Check sheet for the modelled part. Datum: model origin and axes. Units: mm. A direction names the side the tool comes from. Give positions to 0.01 mm unless a question says otherwise; leave off trailing zeros. Order: outer loops, then holes, each group sorted by start corner. A loop starts at its lowest first (then second) coordinate and runs counter-clockwise, first axis right, second up. Notation, with made-up numbers: (76.25, 55) -> (129.25, 55) arc R20 ccw to (129.25, 76) -> close; hole circle Ø10 at (55, -29). An arc over 180 degrees is marked (long way). One line per question, with ' | ' between items. Start each with the question number.
from build123d import *

# Parameters (mm, degrees)
SKETCH1_R           = 2
BOSS_EXTRUDE1_DEPTH = 5
SKETCH4_W           = 1.5
SKETCH4_H           = 7.95
BOSS_EXTRUDE2_DEPTH = 2.5


with BuildPart() as part:
    # Sketch1 → Boss-Extrude1 (new body)
    with BuildSketch(Plane(origin=(0, 0, 0), x_dir=(1, 0, 0), z_dir=(0, 1, 0))):
        with BuildLine():
            Line((-15.567316533, 33.749050158), (15.645012234, 33.749050158))
            ThreePointArc((15.645012234, 33.749050158), (0.03884785, -36.272711642), (-15.567316533, 33.749050158))
        make_face()
        with Locations(Location((-3.21115215, -17.772711642, 0), (0, 0, 270))):
            Circle(SKETCH1_R, mode=Mode.SUBTRACT)
        with Locations(Location((3.28884785, -17.772711642, 0), (0, 0, 270))):
            Circle(SKETCH1_R, mode=Mode.SUBTRACT)
        with BuildLine():
            Line((-14.493890345, 30.38317441), (14.510950609, 30.412564234))
            ThreePointArc((14.510950609, 30.412564234), (25.953877048, 21.309325265), (32.384983632, 8.177288358))
            Line((32.384983632, 8.177288358), (19.014237034, 8.177288358))
            Line((19.014237034, 8.177288358), (19.014237034, -3.272711642))
            Line((19.014237034, -3.272711642), (33.076704924, -3.272711642))
            ThreePointArc((33.076704924, -3.272711642), (24.427207658, -22.122941859), (6.28884785, -32.180023227))
            Line((6.28884785, -32.180023227), (6.28884785, -17.772711642))
            ThreePointArc((6.28884785, -17.772711642), (5.410168194, -15.651391298), (3.28884785, -14.772711642))
            Line((3.28884785, -14.772711642), (-3.21115215, -14.772711642))
            ThreePointArc((-3.21115215, -14.772711642), (-5.332472493, -15.651391298), (-6.21115215, -17.772711642))
            Line((-6.21115215, -17.772711642), (-6.21115215, -32.180023227))
            ThreePointArc((-6.21115215, -32.180023227), (-24.349511958, -22.122941859), (-32.999009223, -3.272711642))
            Line((-32.999009223, -3.272711642), (-3.25, -3.272711642))
            Line((-3.25, -3.272711642), (-3.25, 8.177288358))
            Line((-3.25, 8.177288358), (-32.307287931, 8.177288358))
            ThreePointArc((-32.307287931, 8.177288358), (-25.897276574, 21.283055583), (-14.493890345, 30.38317441))
        make_face(mode=Mode.SUBTRACT)
    extrude(amount=BOSS_EXTRUDE1_DEPTH)

    # Sketch4 → Boss-Extrude2 (add)
    with BuildSketch(Plane(origin=(0, 5, 0), x_dir=(1, 0, 0), z_dir=(0, 1, 0))):
        with Locations((21.065838417, 1.952288358)):
            Rectangle(SKETCH4_W, SKETCH4_H)
        with Locations((-5.488142716, 1.952288358)):
            Rectangle(SKETCH4_W, SKETCH4_H)
    extrude(amount=BOSS_EXTRUDE2_DEPTH)


solid = part.part
1. Cross-section at C-C on z = -18. Record the boundary of the cut face in (x, y), and give its area (3 significant figures).
2. Cross-section at B-B on x = 23.5. Record the boundary of the cut face in (y, z).
3. Cross-section at D-D on x = 9.5. Record the boundary of the cut face in (y, z), and give its area (3 significant figures).
4. Tool access check on faces 1 (the face through (-3.25, 2, -2)), 2 (the face through (20.316, 6, -2)). Record the directions out of +Z, -Z, +X, -X, +Y, -Y that give a thin tool (end or side, any length) a straight path to the whole face; none if there is none.
5. Mould release check, pull along Z, two halves, no side actions. Record for faces 3 (the face through (2.52, 2.46, 19.62)), 4 (the face through (21.816, 6, -2)), 5 (the face through (26, 2, 3.273)), 6 (the face through (0, 2, -33.749)): +Z half, -Z half, draft (parallel to the pull), parting line (faces both ways), or undercut.
6. Go/stop test with flat-tipped pins: pin 1 (4 mm diameter, centred on x = -12, y = 3.5, fed in from +Z) (3 decimals); pin 2 (2 mm diameter, centred on y = 5.5, z = -1.5, fed in from +X); pin 3 (5 mm diameter, centred on x = 3.29, z = 17.77, fed in from -Y); pin 4 (1.5 mm diameter, centred on y = 3.5, z = 27, fed in from +X). Record where each tip stops, or that it passes through.
7. Scan lines: probe 1 along X at (y, z) = (4.5, -1); probe 2 along Z at (x, y) = (-7.5, 3.5); probe 3 along X at (y, z) = (6.75, -0.5). Record each from-to range of solid material in increasing order.
8. Cross-section at A-A on y = 2.75. Record the boundary of the cut face in (x, z).
Response values:
1) outline: (-32.26, 0) -> (-28.22, 0) -> (-28.22, 5) -> (-32.26, 5) -> close; (28.3, 0) -> (32.34, 0) -> (32.34, 5) -> (28.3, 5) -> close | area: 40.5 mm²
2) outline: (0, -28.76) -> (5, -28.76) -> (5, -24.04) -> (0, -24.04) -> close; (0, -8.18) -> (5, -8.18) -> (5, 3.27) -> (0, 3.27) -> close; (0, 23.08) -> (5, 23.08) -> (5, 27.81) -> (0, 27.81) -> close
3) outline: (0, -33.75) -> (5, -33.75) -> (5, -30.41) -> (0, -30.41) -> close; (0, 31.4) -> (5, 31.4) -> (5, 35.03) -> (0, 35.03) -> close | area: 34.9 mm²
4) face 1: +Y, -Y | face 2: +Z, -Z, +Y
5) face 3: undercut | face 4: draft | face 5: undercut | face 6: -Z half
6) pin 1: stops at z = 34.875 | pin 2: stops at x = 36.79 | pin 3: stops at y = 0 | pin 4: stops at x = 25.26
7) probe 1: x = -36.71 to -3.25, 19.01 to 36.79 | probe 2: z = -33.75 to -30.39, -8.18 to 3.27, 31.91 to 35.49 | probe 3: x = -6.24 to -4.74, 20.32 to 21.82
8) outline: (-15.57, -33.75) -> (15.65, -33.75) arc R36.75 ccw (long way) to start; hole (-33, 3.27) -> (-3.25, 3.27) -> (-3.25, -8.18) -> (-32.31, -8.18) arc R33.25 ccw to (-14.49, -30.38) -> (14.51, -30.41) arc R33.25 ccw to (32.38, -8.18) -> (19.01, -8.18) -> (19.01, 3.27) -> (33.08, 3.27) arc R33.25 ccw to (6.29, 32.18) -> (6.29, 17.77) arc R3 cw to (3.29, 14.77) -> (-3.21, 14.77) arc R3 cw to (-6.21, 17.77) -> (-6.21, 32.18) arc R33.25 ccw to start; hole circle Ø4 at (-3.21, 17.77); hole circle Ø4 at (3.29, 17.77)
